Design review of the part built by this model. Coordinates are the model's own, in mm. A direction names the side the tool comes from. Give positions to 0.01 mm unless a question says otherwise; leave off trailing zeros. Write each loop counter-clockwise with the first axis right and the second up, starting at its lowest first coordinate (ties: lowest second). Pieces come first, ordered by that corner, then holes. Notation, with made-up numbers: (5, -14) -> (14, -14) arc R21 ccw to (14, 14) -> close; hole circle Ø3 at (9.25, -6.5). An arc over 180 degrees is marked (long way). Use CSV: the item, a comma, the result in double quotes.
```python
from build123d import *

# Parameters (mm, degrees)
RESSALTO_EXTRUS_O1_DEPTH = 19
FILETE1_R                = 0.2
ESBO_O2_R                = 1.0922
RESSALTO_EXTRUS_O2_DEPTH = 4.76
ESBO_O3_R                = 1.0922
CORTE_EXTRUS_O1_DEPTH    = 4.76


with BuildPart() as part:
    # Esboço1 → Ressalto-extrusão1 (new body)
    with BuildSketch(Plane(origin=(0, 0, 0), x_dir=(1, 0, 0), z_dir=(0, 1, 0))):
        Polygon((2.748187281, 0), (1.374093641, 2.38), (-1.374093641, 2.38), (-2.748187281, 0), (-1.374093641, -2.38), (1.374093641, -2.38), align=None)
    extrude(amount=RESSALTO_EXTRUS_O1_DEPTH)

    # Filete1
    filete1_edges = [part.edges().sort_by_distance(p)[0] for p in [
        (0, 19, -2.38),
        (-2.061140461, 19, -1.19),
        (-2.061140461, 19, 1.19),
        (0, 19, 2.38),
        (2.061140461, 19, 1.19),
        (0, 0, 2.38),
        (-2.061140461, 0, 1.19),
        (-2.061140461, 0, -1.19),
        (2.061140461, 19, -1.19),
        (0, 0, -2.38),
        (2.061140461, 0, -1.19),
        (2.061140461, 0, 1.19),
    ]]
    fillet(filete1_edges, radius=FILETE1_R)

    # Esboço2 → Ressalto-extrusão2 (add)
    with BuildSketch(Plane.XZ):
        Circle(ESBO_O2_R)
    extrude(amount=RESSALTO_EXTRUS_O2_DEPTH)

    # Esboço3 → Corte-extrusão1 (cut)
    with BuildSketch(Plane(origin=(0, 19, 0), x_dir=(1, 0, 0), z_dir=(0, 1, 0))):
        Circle(ESBO_O3_R)
    extrude(amount=-CORTE_EXTRUS_O1_DEPTH, mode=Mode.SUBTRACT)


solid = part.part
```
(1) Mouldability with a two-part tool opening along X and no side actions: class faces 3 (the face through (-2.021, 0.06, -1.145)), 4 (the face through (0, -4.76, 0)), 5 (the face through (1.04, 16.65, -0.33)), 6 (the face through (2, 0.06, -1.18)) as +X half, -X half, draft (parallel to the pull), parting line (faces both ways), or undercut.
Established:
face 3,"-X half"
face 4,"draft"
face 5,"undercut"
face 6,"+X half"
(2) Clearance check with flat-ended pins moving along their axes: pin 1 (1 mm diameter, centred on y = 14.5, z = 2, fed in from -X); pin 2 (2 mm diameter, centred on y = 15, z = 0.5, fed in from +X). State where each tip first meets the part, or that it passes through.
Established:
pin 1,"stops at x = -1.88"
pin 2,"stops at x = 2.75"
(3) Tool access review of faces 1 (the face through (1, 0, -1)), 2 (the face through (2.05, 9.37, 1.21)): name each direction out of +Z, -Z, +X, -X, +Y, -Y from which nothing blocks a thin tool from reaching the whole face with its end or side.
Established:
face 1,"-Y"
face 2,"+Z, +X, +Y, -Y"
(4) Take a section at C-C (x = -0.7). Write out the cut boundary in (y, z).
Established:
outline,"(-4.76, -0.84) -> (0, -0.84) -> (0, -2.18) arc R0.2 ccw to (0.2, -2.38) -> (18.8, -2.38) arc R0.2 ccw to (19, -2.18) -> (19, -0.84) -> (14.24, -0.84) -> (14.24, 0.84) -> (19, 0.84) -> (19, 2.18) arc R0.2 ccw to (18.8, 2.38) -> (0.2, 2.38) arc R0.2 ccw to (0, 2.18) -> (0, 0.84) -> (-4.76, 0.84) -> close"
(5) Take a section at A-A (y = 15.5). Write out the cut boundary in (x, z), then the cut area to 3 significant figures.
Established:
outline,"(-2.75, 0) -> (-1.37, -2.38) -> (1.37, -2.38) -> (2.75, 0) -> (1.37, 2.38) -> (-1.37, 2.38) -> close; hole circle Ø2.18 at (0, 0)"
area,"15.9 mm2"
(6) Take a section at D-D (y = -0.5). Write out the cut boundary in (x, z).
Established:
outline,"circle Ø2.18 at (0, 0)"
(7) Take a section at B-B (y = 12.5). Write out the cut boundary in (x, z).
Established:
outline,"(-2.75, 0) -> (-1.37, -2.38) -> (1.37, -2.38) -> (2.75, 0) -> (1.37, 2.38) -> (-1.37, 2.38) -> close"
(8) For line 1 along Z through (x, y) = (0, 17.75); line 2 along Y through (x, z) = (1.3, -0.75); line 3 along Y through (x, z) = (0.45, -0.5), list the stretches that pass through material, from the lowest coordinate up. Write a range as [from, to].
Established:
line 1,"z = [-2.38, -1.09], [1.09, 2.38]"
line 2,"y = [0, 19]"
line 3,"y = [-4.76, 14.24]"
